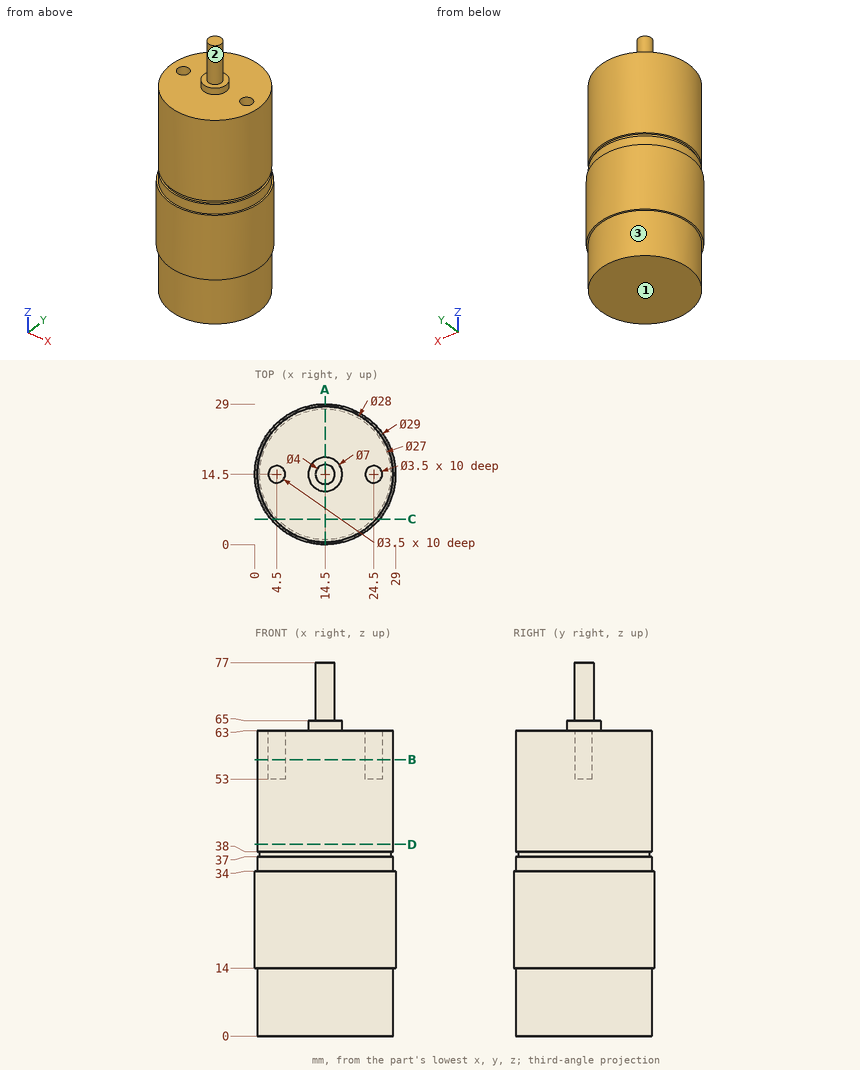
Can you work these out from the drawing? Everything is in mm from the part's minimum corner. A direction names the side the tool comes from. Give positions to 0.01 mm unless a question says otherwise; leave off trailing zeros. Loops run counter-clockwise (first coordinate to the right, second up) from the corner with the lowest first, then second, coordinate; pieces in that order, holes last. Notation, with made-up numbers: M 59.5,78 L 90.5,78 A22 ccw 90.5,107 Z; hole C 52,67 d2. An arc over 180 degrees is marked long. Use CSV: the item, a comma, the result in double quotes. Start each with the question number.
1. Imagine slicing it at A-A, the plane x = 14.5. Write out the boundary of the cut face in (y, z).
2. On a 3-axis mill with a long thin cutter (end or side, diameter ignored), from which of +Z, -Z, +X, -X, +Y, -Y can I reach the whole of each face in a straight line? I mean the marked faces 1, 2 and 3. Say none if no direction works.
3. Imagine slicing it at B-B, the plane z = 57. Write out the boundary of the cut face in (x, y).
4. Imagine slicing it at C-C, the plane y = 5.25. Write out the boundary of the cut face in (x, z).
5. For P1, Ø4, axis at x = 15.5, z = 36.5, coming from the +Y side; P2, Ø8, axis at y = 7, z = 12, coming from the -X side; P3, Ø2, axis at x = 24.5, y = 14.5, coming from the +Z side, each with a flat end and sliding along its axis, tell me the tip position at first contact or that it passes through.
6. Imagine slicing it at D-D, the plane z = 39.5. Write out the boundary of the cut face in (x, y).
7. If I drill on L1, parallel to Z at x = 23.5, y = 4.75; L2, parallel to Y at x = 24.5, z = 57.25; L3, parallel to X at y = 21.5, z = 58.5, over which ranges is the centre line in solid material (lowest first)?
Response values:
1,outline,"M 0,14 L 0.5,14 L 0.5,0 L 28.5,0 L 28.5,14 L 29,14 L 29,34 L 28.5,34 L 28.5,37 L 28,37 L 28,38 L 28.5,38 L 28.5,63 L 18,63 L 18,65 L 16.5,65 L 16.5,77 L 12.5,77 L 12.5,65 L 11,65 L 11,63 L 0.5,63 L 0.5,38 L 1,38 L 1,37 L 0.5,37 L 0.5,34 L 0,34 Z"
2,face 1,"-Z, +X, -X, +Y, -Y"
2,face 2,"+Z"
2,face 3,"-Z"
3,outline,"C 14.5,14.5 d28; hole C 4.5,14.5 d3.5; hole C 24.5,14.5 d3.5"
4,outline,"M 3.33,14 L 3.99,14 L 3.99,0 L 25.01,0 L 25.01,14 L 25.67,14 L 25.67,34 L 25.01,34 L 25.01,37 L 24.33,37 L 24.33,38 L 25.01,38 L 25.01,63 L 3.99,63 L 3.99,38 L 4.67,38 L 4.67,37 L 3.99,37 L 3.99,34 L 3.33,34 Z"
5,P1,"y = 28.5"
5,P2,"x = 0.57"
5,P3,"z = 53"
6,outline,"C 14.5,14.5 d28"
7,L1,"0 to 63"
7,L2,"4.7 to 12.75, 16.25 to 24.3"
7,L3,"2.38 to 26.62"
